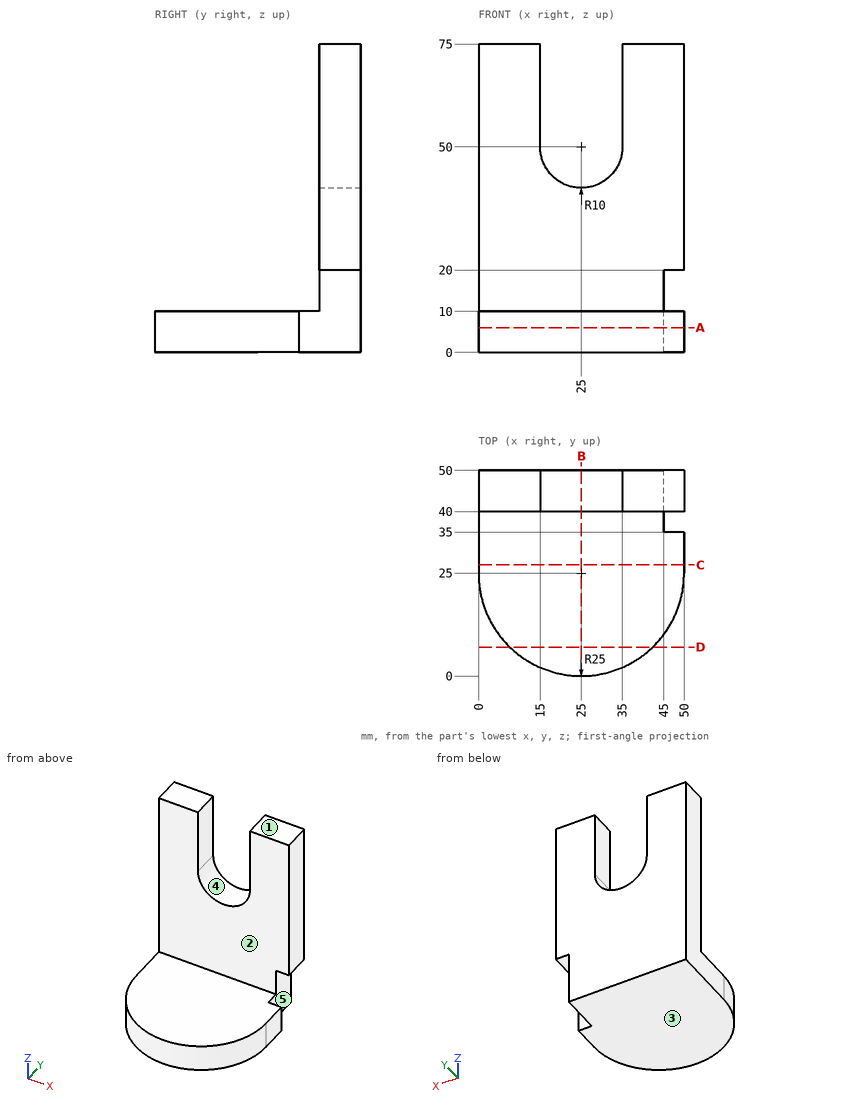
Check sheet for the drawn part. Datum: minimum x, y, z corner. Units: mm. A direction names the side the tool comes from. Give positions to 0.01 mm unless a question says otherwise; leave off trailing zeros. Write each loop counter-clockwise with the first axis right and the second up, starting at its lowest first coordinate (ties: lowest second). Pieces come first, ordered by that corner, then holes. Notation, with made-up numbers: (16, 72.5) - (52, 72.5) arc R13 cw to (52, 78.5) - close; hole circle Ø4 at (64.25, 30). An arc over 180 degrees is marked (long way). Put each result on its own line as item: value.
1. Set-up check for the marked faces 1 and 2: record each of +Z, -Z, +X, -X, +Y, -Y from which the full face is reachable in a straight line by a thin tool's end or side.
Ans:
face 1: +Z, +X, -X, +Y, -Y
face 2: +Z, +X, -X, -Y
2. Sectioned sample at A-A, the plane z = 6. Enter the section's corners in (x, y), plus the area to 3 significant figures.
Ans:
outline: (0, 25) arc R25 ccw to (50, 25) - (50, 35) - (45, 35) - (45, 50) - (0, 50) - close
area: 2,160 mm²
3. Go/stop test with flat-tipped pins: pin 1 (5.5 mm diameter, centred on x = 47, y = 44.5, fed in from -Z); pin 2 (2 mm diameter, centred on x = 5.5, y = 25.5, fed in from +Z); pin 3 (25 mm diameter, centred on x = 14, z = 47, fed in from -Y); pin 4 (4.5 mm diameter, centred on y = 40, z = 14.5, fed in from +X). Record where each tip stops, or that it passes through.
Ans:
pin 1: stops at z = 0
pin 2: stops at z = 10
pin 3: stops at y = 40
pin 4: stops at x = 45
4. Draft check along X on the marked faces 3, 4 and 5. Enter one of: +X half, -X half, draft (parallel to the pull), parting line (faces both ways), or undercut.
Ans:
face 3: draft
face 4: undercut
face 5: +X half
5. Sectioned sample at B-B, the plane x = 25. Enter the section's corners in (y, z).
Ans:
outline: (0, 0) - (50, 0) - (50, 40) - (40, 40) - (40, 10) - (0, 10) - close
6. Thickness scan on line 1 (X direction, y = 46.5, z = 70); line 2 (Z direction, x = 7, y = 12); line 3 (Y direction, x = 18, z = 36.5). Record the ranges inside material, lowest first.
Ans:
line 1: x = 0 to 15, 35 to 50
line 2: z = 0 to 10
line 3: y = 40 to 50
7. Sectioned sample at D-D, the plane y = 7. Enter the section's corners in (x, z).
Ans:
outline: (7.65, 0) - (42.35, 0) - (42.35, 10) - (7.65, 10) - close
8. Sectioned sample at C-C, the plane y = 27. Enter the section's corners in (x, z), plus the area to 3 significant figures.
Ans:
outline: (0, 0) - (50, 0) - (50, 10) - (0, 10) - close
area: 500 mm²
